The listing builds one solid part. Answer for the finished solid, in the listing's coordinates (mm). A direction names the side the tool comes from. Round coordinates to 2 decimals unless told otherwise and drop trailing zeros. Loops run counter-clockwise (first coordinate to the right, second up) from the corner with the lowest first, then second, coordinate; pieces in that order, holes last. Notation, with made-up numbers: M 28.25,30.25 L 78.25,30.25 A14 cw 78.25,41.25 Z; hole C 27,-7.5 d4. An arc over 180 degrees is marked long. Answer as a JSON object with one key per item and string values.
Autodesk Inventor part; units mm, degrees
ref_plane "YZ Plane" through (0, 0, 0) normal (1, 0, 0) x (0, 1, 0)
ref_plane "XZ Plane" through (0, 0, 0) normal (0, 1, 0) x (-1, 0, 0)
ref_plane "XY Plane" through (0, 0, 0) normal (0, 0, 1) x (1, 0, 0)
sketch "Sketch1" plane through (0, 0, 0) normal (0, 0, 1) x (1, 0, 0)
  line L0 (-46, -50) -> (46, -50)
  line L1 (46, -50) -> (46, 50)
  line L2 (46, 50) -> (-46, 50)
  line L3 (-46, 50) -> (-46, -50)
  line L4 (-46, -50) -> (46, 50) construction
  line L5 (46, -50) -> (-46, 50) construction
  point P0 (0, 0)
  dimension "d154" = 92
  dimension "d155" = 100
extrude "Plate5" add sketch "Sketch1" along normal blind 2
sketch "Sketch7" plane through (-44, -50, 0) normal (-1, 0, 0) x (0, -1, 0)
  line L0 (-100, 0) -> (0, 0)
  line L1 (0, 0) -> (0, 94)
  line L2 (0, 94) -> (-100, 94)
  line L3 (-100, 94) -> (-100, 0)
edge flange "Flange3" height 94 angle 90 thickness 2 bend radius 2.75 thickness toward (-1, 0, 0) relief round relief width 2 relief depth 1 edges at (-46, 0, 2) wall of the first edge with corners at (-44, 50, 0) (-44, -50, 0) (-44, -50, 94) (-44, 50, 94)
bend "Bend3"
corner "Corner3"
sketch "Sketch8" plane through (0, 0, 2) normal (0, 0, 1) x (1, 0, 0)
  line L0 (46, 50) -> (46, -50)
  line L1 (-41.25, 50) -> (46, 50)
  line L2 (31.375, 45) -> (-26.625, 45)
  line L3 (-26.625, 45) -> (-26.625, -13)
  line L4 (-26.625, -13) -> (31.375, -13)
  line L5 (31.375, -13) -> (31.375, 45)
  line L6 (31.375, 45) -> (-26.625, -13) construction
  line L7 (-26.625, 45) -> (31.375, -13) construction
  point P0 (0, 0)
  point P1 (2.375, 16)
  point P2 (2.375, 50)
  dimension "d167" = 58
  dimension "d168" = 58
  dimension "d169" = 5
extrude "Cut1" cut sketch "Sketch8" against normal blind 2
properties part number "TZS 1652 FDS Central tube wall" material "Stainless Steel"
Item 1: Which of the six approach directions +Z, -Z, +X, -X, +Y, -Y give full straight-line access (tool end or side, diameter ignored) to faces 1 (the face through (-44, -1, 49)), 2 (the face through (2, -22, 0))?
Values follow:
{"face 1": "+Z, +X, +Y, -Y", "face 2": "-Z, +X, -X, +Y, -Y"}
Item 2: The part is cut by section B-B (x = 30). Give the vertices of the cut face in (y, z), then the cut area to 3 significant figures.
Values follow:
{"outline": "M -50,0 L -13,0 L -13,2 L -50,2 Z; M 45,0 L 50,0 L 50,2 L 45,2 Z", "area": "84.0 mm^2"}
Item 3: The part is cut by section D-D (z = 25.5). Give the vertices of the cut face in (x, y), then the cut area to 3 significant figures.
Values follow:
{"outline": "M -46,-50 L -44,-50 L -44,50 L -46,50 Z", "area": "200 mm^2"}
Item 4: Straight lines are drawn through the part: line 1 (X direction, y = 12, z = 28); line 2 (Z direction, x = -31.5, y = 42); line 3 (X direction, y = 22, z = 4). For each, find the intervals that lie inside material, in ascending order.
Values follow:
{"line 1": "-46 to -44", "line 2": "0 to 2", "line 3": "-45.94 to -43.9"}
Item 5: The part is cut by section A-A (y = 37). Give the vertices of the cut face in (x, z) (3 decimals), then the cut area to 3 significant figures.
Values follow:
{"outline": "M -46,4.75 A4.75 ccw -41.25,0 L -26.625,0 L -26.625,2 L -41.25,2 A2.75 cw -44,4.75 L -44,94 L -46,94 Z; M 31.375,0 L 46,0 L 46,2 L 31.375,2 Z", "area": "249 mm^2"}
Item 6: The part is cut by section C-C (y = -35.5). Give the vertices of the cut face in (x, z).
Values follow:
{"outline": "M -46,4.75 A4.75 ccw -41.25,0 L 46,0 L 46,2 L -41.25,2 A2.75 cw -44,4.75 L -44,94 L -46,94 Z"}
Item 7: Flat-ended cylindrical pins translate along their axes: P1, Ø4, axis at x = 1.5, y = -24.5, coming from the +Z side; P2, Ø1.5, axis at y = 11, z = 32, coming from the +X side; P3, Ø0.6, axis at y = 29.5, z = 1, coming from the -X side. Find the tip coordinate at first contact, or state that the pin passes through.
Values follow:
{"P1": "z = 2", "P2": "x = -44", "P3": "x = -44.51"}
